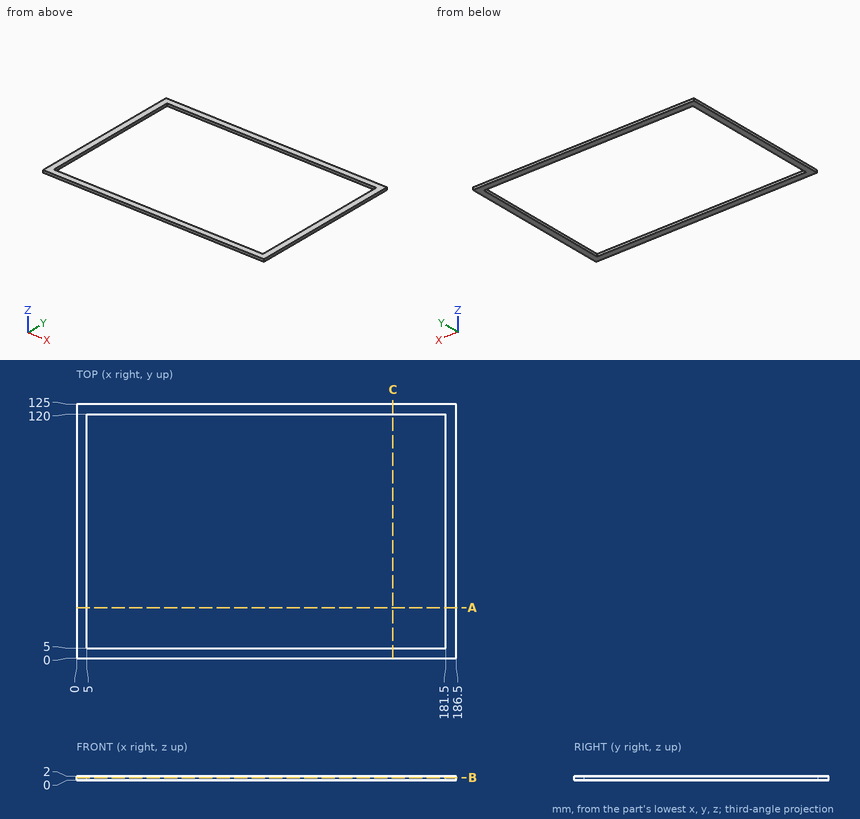
Job drawing, mm, ordinate dimensions from the low corner. One solid piece. Give positions to 0.01 mm unless a question says otherwise; leave off trailing zeros. Write each loop counter-clockwise with the first axis right and the second up, starting at its lowest first coordinate (ties: lowest second). Pieces come first, ordered by that corner, then holes. Notation, with made-up numbers: M 19.5,79.5 L 33.5,79.5 A16 cw 33.5,86.5 Z; hole C 71.5,89.25 d5. An arc over 180 degrees is marked long. One line per item, written item: value. Start each with the question number.
Q1. Saw through at B-B, the plane z = 1.35. Write the cut outline in (x, y), plus the area to 4 significant figures.
Q2. Saw through at A-A, the plane y = 25. Write the cut outline in (x, z), plus the area to 3 significant figures.
Q3. Saw through at C-C, the plane x = 155.5. Write the cut outline in (y, z).
Q4. Probe probe 1 along X at (y, z) = (54, 1.05); probe 2 along Y at (x, z) = (61.5, 0.45). List the from-to ranges inside material, lowest first. Write a range as [from, to].
Output values:
1. outline: M 0,0 L 186.5,0 L 186.5,125 L 0,125 Z; hole M 5,5 L 181.5,5 L 181.5,120 L 5,120 Z
1. area: 3,015 mm²
2. outline: M 0,0 L 5,0 L 5,2 L 0,2 Z; M 181.5,0 L 186.5,0 L 186.5,2 L 181.5,2 Z
2. area: 20.0 mm²
3. outline: M 0,0 L 5,0 L 5,2 L 0,2 Z; M 120,0 L 125,0 L 125,2 L 120,2 Z
4. probe 1: x = [0, 5], [181.5, 186.5]
4. probe 2: y = [0, 5], [120, 125]
